CAD build for the part. Positions are in the model's coordinates, mm. Face numbers are marked on the shaded views. A direction names the side the tool comes from. Coordinates: 2 decimals unless noted, no trailing zeros.
1) Pin check, flat tips, straight feed: pin 1 Ø16.5 at (x, y) = (24, 11.5) entering from +Z; pin 2 Ø8 at (x, y) = (7, 7) entering from -Z; pin 3 Ø9 at (y, z) = (13.5, -0.5) entering from -X. Stop position of each tip, or through.
2) Which spindle directions (+Z, -Z, +X, -X, +Y, -Y) get a long thin tool onto all of the face, cutting with end or side? Do the marked faces 1, 2 and 3. Say none if no direction does.
3) Wall check: line 1 along X through (y, z) = (28, 0); line 2 along X through (y, z) = (8, 0); line 3 along Z through (x, y) = (29.5, 11). Give the ranges that are in metal, low to high.
4) Saw through at A-A, the plane y = 9. Give the number of separate pieces and of enclosed holes in the cut face, and give its area (3 significant figures).
5) Two-plate mould, pull along Z, no slides. Class the marked faces 4, 5 and 6: +Z half, -Z half, draft (parallel to the pull), parting line (faces both ways), or undercut.
```python
from build123d import *

# Parameters (mm, degrees)
SKETCH1_R               = 17
SKETCH1_R_2             = 15
BOSS_EXTRUDE1_DEPTH     = 40
SKETCH2_R               = 26
SKETCH2_R_2             = 15
BOSS_EXTRUDE2_DEPTH     = 15
FILLET1_R               = 10
BOSS_EXTRUDE4_REACH     = 56.331
SKETCH3_R               = 5
SKETCH3_R_2             = 3
CUT_EXTRUDE1_START      = -38
SKETCH4_R               = 3
CUT_EXTRUDE1_DEPTH      = 38
SKETCH5_R               = 15
BOSS_EXTRUDE5_DEPTH     = 2
BOSS_EXTRUDE10_START    = -40
SKETCH13_W              = 15
SKETCH13_H              = 36
BOSS_EXTRUDE10_DEPTH    = 20
CUT_EXTRUDE4_DEPTH      = 49.702222157
CUT_EXTRUDE4_DEPTH_BACK = 49.702222157
SKETCH14_W              = 15
SKETCH14_H              = 36
SKETCH15_W              = 15
SKETCH15_H              = 36
BOSS_EXTRUDE11_DEPTH    = 2


with BuildPart() as part:
    # Sketch1 → Boss-Extrude1 (new body)
    with BuildSketch(Plane(origin=(0, 0, 0), x_dir=(1, 0, 0), z_dir=(0, 1, 0))):
        with Locations(Location((0, 0, 0), (0, 0, 270))):
            Circle(SKETCH1_R)
        with Locations(Location((0, 0, 0), (0, 0, 270))):
            Circle(SKETCH1_R_2, mode=Mode.SUBTRACT)
    extrude(amount=BOSS_EXTRUDE1_DEPTH)

    # Sketch2 → Boss-Extrude2 (add)
    with BuildSketch(Plane.XZ):
        with Locations(Location((0, 0, 0), (0, 0, 270))):
            Circle(SKETCH2_R)
        with Locations(Location((0, 0, 0), (0, 0, 90))):
            Circle(SKETCH2_R_2, mode=Mode.SUBTRACT)
    extrude(amount=-BOSS_EXTRUDE2_DEPTH)

    # Fillet1
    # the kernel refuses this fillet: 10 mm, written as the material it adds along each edge
    with BuildSketch(Plane(origin=(0, 15, 0), x_dir=(0, 0, 1), z_dir=(1, 0, 0))) as fillet1_piece_1:
        with BuildLine():
            CenterArc((27, -9.949874371), FILLET1_R, 95.739170477, 84.260829523)
            Line((17, -9.949874371), (16.8, -9.949874371))
            Line((16.8, -9.949874371), (16.8, 0))
            Line((16.8, 0), (17, 0.2))
            ThreePointArc((17, 0.2), (21.5, 0.2), (25.98, 0.198997487))
            Line((25.98, 0.198997487), (26, 0))
        make_face()
    revolve(axis=Axis((0, 15, 0), (0, -1, 0)))

    # Fillet2: read off the stored shape, not the designer's step
    # Fillet2 outline → Fillet2 (revolve, cut)
    with BuildSketch(Plane.XY):
        with BuildLine():
            Line((25.998200588, 18.630262041), (19.25, 18.630262041))
            ThreePointArc((19.25, 18.630262041), (24.206637205, 9.888353044), (25.998200588, 0))
            Line((25.998200588, 0), (25.998200588, 18.630262041))
        make_face()
    revolve(axis=Axis((0, 0, 0), (0, 1, 0)), mode=Mode.SUBTRACT)

    # Fillet2 2 outline → Fillet2 2 (revolve, cut)
    with BuildSketch(Plane.XY):
        with BuildLine():
            Line((26, 0), (26, 15))
            ThreePointArc((26, 15), (25.999100287, 15.000090466), (25.998200582, 15.000181013))
            Line((25.998200582, 15.000181013), (25.998200588, 0))
            Line((25.998200588, 0), (26, 0))
        make_face()
    revolve(axis=Axis((0, 0, 0), (0, 1, 0)), mode=Mode.SUBTRACT)

    # Boss-Extrude4: up to this face of the body (flat: up to its plane)
    boss_extrude4_end = Plane(part.part.faces().sort_by_distance((0, 40, -16.519167389))[0])
    # Sketch3 → Boss-Extrude4 (add, up to the picked face)
    with BuildSketch(Plane.XZ, mode=Mode.PRIVATE) as boss_extrude4_sk1:
        with Locations((-20.499100294, 0)):
            Circle(SKETCH3_R)
        with Locations(Location((-20.499100294, 0, 0), (0, 0, 298.480209609))):
            Circle(SKETCH3_R_2, mode=Mode.SUBTRACT)
    boss_extrude4_tool1 = split(extrude(boss_extrude4_sk1.sketch, amount=-BOSS_EXTRUDE4_REACH, mode=Mode.PRIVATE), bisect_by=boss_extrude4_end, keep=Keep.BOTH, mode=Mode.PRIVATE)
    add(boss_extrude4_tool1.solids().sort_by(Axis((-25.357679, 0, 0), (0, 1, 0)))[0])

    # Sketch4 → Cut-Extrude1 (cut)
    with BuildSketch(Plane(origin=(0, 40, 0), x_dir=(1, 0, 0), z_dir=(0, 1, 0)).offset(CUT_EXTRUDE1_START)):
        with Locations(Location((-20.499100294, 0, 0), (0, 0, 270))):
            Circle(SKETCH4_R)
    extrude(amount=CUT_EXTRUDE1_DEPTH, mode=Mode.SUBTRACT)

    # Sketch5 → Boss-Extrude5 (add)
    with BuildSketch(Plane.XZ):
        with Locations(Location((0, 0, 0), (0, 0, 270))):
            Circle(SKETCH5_R)
    extrude(amount=-BOSS_EXTRUDE5_DEPTH)

    # Sketch13 → Boss-Extrude10 (add)
    with BuildSketch(Plane(origin=(0, 40, 0), x_dir=(1, 0, 0), z_dir=(0, 1, 0)).offset(BOSS_EXTRUDE10_START)):
        Polygon((17, 0), (17, 20), (36, 20), (36, -20), (16.610431475, -20), align=None)
        with Locations((26.5, 0)):
            Rectangle(SKETCH13_W, SKETCH13_H, mode=Mode.SUBTRACT)
    extrude(amount=BOSS_EXTRUDE10_DEPTH)

    # Sketch14 → Cut-Extrude4 (cut, two sides: drawn at the far end of the back side and taken through both)
    with BuildSketch(Plane(origin=(0, 20, 0), x_dir=(1, 0, 0), z_dir=(0, 1, 0)).offset(-CUT_EXTRUDE4_DEPTH_BACK)):
        with Locations((26.5, 0)):
            Rectangle(SKETCH14_W, SKETCH14_H)
    extrude(amount=CUT_EXTRUDE4_DEPTH + CUT_EXTRUDE4_DEPTH_BACK, mode=Mode.SUBTRACT)

    # Sketch15 → Boss-Extrude11 (add)
    with BuildSketch(Plane.XZ):
        with Locations((26.5, 0)):
            Rectangle(SKETCH15_W, SKETCH15_H)
    extrude(amount=-BOSS_EXTRUDE11_DEPTH)


solid = part.part
```
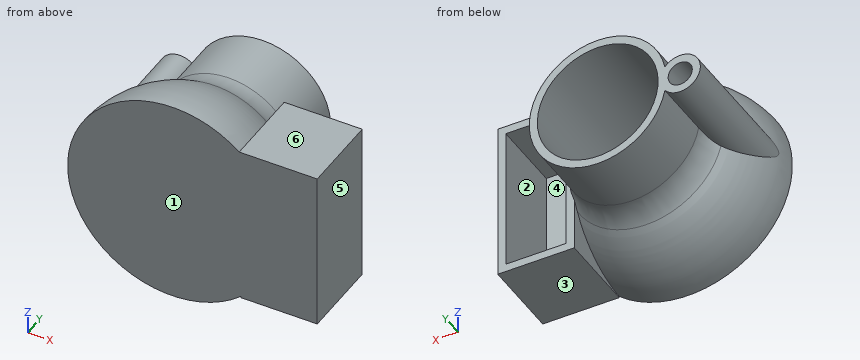
Data:
1. pin 1: stops at z = 20
1. pin 2: stops at z = -25.32
1. pin 3: stops at x = -25.5
2. face 1: +Z, -Z, +X, -X, -Y
2. face 2: +Y
2. face 3: -Z, +X, +Y, -Y
3. line 1: x = -25.5 to -23.5, -17.5 to -15, 15 to 17
3. line 2: x = -25.5 to -23.5, -17.5 to -15, 15 to 19, 34 to 36
3. line 3: z = -20 to -18, 18 to 20
4. separate pieces: 1
4. enclosed holes: 3
4. area: 1,190 mm2
5. face 4: undercut
5. face 5: draft
5. face 6: +Z half
